Model file for the job. Use its own axes, mm. Round coordinates to 2 decimals unless told otherwise and drop trailing zeros. Order: outer loops, then holes, each group sorted by start corner. A loop starts at its lowest first (then second) coordinate and runs counter-clockwise, first axis right, second up. Notation, with made-up numbers: M -21.75,-7.75 L 21.25,-7.75 A16 cw 21.25,18.25 Z; hole C 57.5,15 d6. An arc over 180 degrees is marked long. Return JSON: item names as keys, results as strings. Group by question number.
Item 1: Slice it at A-A on z = 0.35. Write the cut outline in (x, y) (3 decimals), then the cut area to 3 significant figures.
Item 2: Probe line 1 along X through (y, z) = (0.25, 0.2); line 2 along Y through (x, z) = (5.5, 0.35); line 3 along X through (y, z) = (-2.25, 0.7). List the from-to ranges inside material, lowest first.
Item 3: Slice it at B-B on y = -3.25. Write the cut outline in (x, z) (3 decimals).
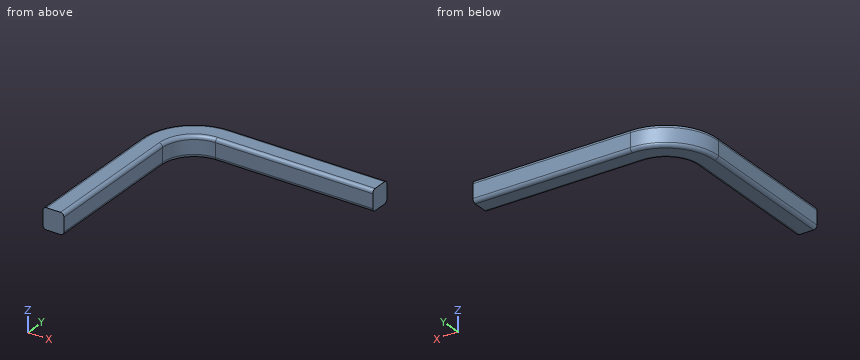
Autodesk Inventor part; units mm, degrees
ref_plane "YZ Plane" through (0, 0, 0) normal (1, 0, 0) x (0, 1, 0)
ref_plane "XZ Plane" through (0, 0, 0) normal (0, 1, 0) x (-1, 0, 0)
ref_plane "XY Plane" through (0, 0, 0) normal (0, 0, 1) x (1, 0, 0)
sketch "Sketch1" plane through (0, 0, 0) normal (0, 0, 1) x (1, 0, 0)
  line L0 (7.62, 2.413) -> (1.905, 2.413)
  line L1 (0, 0.508) -> (0, 0)
  line L2 (0.762, 0) -> (0.762, 0.508)
  line L3 (1.905, 1.651) -> (7.62, 1.651)
  arc A0 (1.905, 1.651) -> (0.762, 0.508) centre (1.905, 0.508) ccw
  arc A1 (1.905, 2.413) -> (0, 0.508) centre (1.905, 0.508) ccw
  line L4 (7.62, 2.413) -> (7.62, 1.651)
  line L5 (0.762, 0) -> (0, 0)
  line L6 (0.762, -4.7752) -> (0, -4.7752)
  line L7 (0, -4.7752) -> (0, 0)
  line L8 (0, 0) -> (0.762, 0)
  line L9 (0.762, 0) -> (0.762, -4.7752)
  point P0 (0, 2.413)
  dimension "d0" = 7.62
  dimension "d1" = 0.762
  dimension "d2" = 1.143
  dimension "d3" = 1.905
  dimension "d4" = 2.413
  dimension "d5" = 4.7752
extrude "Extrusion1" add sketch "Sketch1" along normal blind 0.762
fillet "Fillet2" radius 0.127 8 edges at (1.0968, 1.3162, 0.762) (4.7625, 1.651, 0.762) (0.558, 1.855, 0.762) (4.7625, 2.413, 0.762) (0.558, 1.855, 0) (4.7625, 2.413, 0) (1.0968, 1.3162, 0) (4.7625, 1.651, 0)
properties part number "90d pin_header"
Output values:
{
 "1": {"outline": "M 0,-4.775 L 0.762,-4.775 L 0.762,0.508 A1.143 cw 1.905,1.651 L 7.62,1.651 L 7.62,2.413 L 1.905,2.413 A1.905 ccw 0,0.508 Z", "area": "10.2 mm²"},
 "2": {"line 1": "0 to 0.76", "line 2": "1.65 to 2.41", "line 3": "0.02 to 0.74"},
 "3": {"outline": "M 0,0.127 A0.127 ccw 0.127,0 L 0.635,0 A0.127 ccw 0.762,0.127 L 0.762,0.635 A0.127 ccw 0.635,0.762 L 0.127,0.762 A0.127 ccw 0,0.635 Z"}
}
